```python
from build123d import *

# Parameters (mm, degrees)
SKETCH1_W                        = 69.85
SKETCH1_H                        = 838.2
BASE_FLANGE1_DEPTH               = 3.2639
EDGE_FLANGE2_STRIP_W             = 15.5956
EDGE_FLANGE2_STRIP_H             = 3.2639
EDGE_FLANGE2_STRIP_CUT_DEPTH     = 838.2
EDGE_FLANGE2_STRIP_2_W           = 15.5956
EDGE_FLANGE2_STRIP_2_H           = 3.2639
EDGE_FLANGE2_STRIP_CUT_2_DEPTH   = 838.2
EDGE_FLANGE2_DEPTH               = 838.2
EDGE_FLANGE2_BEND_DEPTH          = 838.2
SKETCH23_W                       = 101.6
SKETCH23_H                       = 34.925
BOSS_EXTRUDE1_DEPTH              = 3.2639
SKETCH24_W                       = 101.6
SKETCH24_H                       = 34.925
BOSS_EXTRUDE2_DEPTH              = 3.2639
SKETCH32_W                       = 88.9
SKETCH32_H                       = 34.925
BOSS_EXTRUDE3_DEPTH              = 3.2639
BOSS_EXTRUDE4_START              = -3.2639
SKETCH33_W                       = 88.9
SKETCH33_H                       = 34.925
BOSS_EXTRUDE4_DEPTH              = 3.2639
F_10_0_1935_DIAMETER_HOLE2_D     = 4.9149
LPATTERN2_COUNT                  = 4
LPATTERN2_PITCH                  = 155.575
F_25_64_0_39063_DIAMETER_HOLE1_D = 9.922002
F_10_0_1935_DIAMETER_HOLE3_D     = 4.9149
FILLET2_R                        = 6.35


# Sheet-metal steps are written as plain solids
with BuildPart() as part:
    # Sketch1 → Base-Flange1 (new body)
    with BuildSketch(Plane(origin=(0, 0, 0), x_dir=(1, 0, 0), z_dir=(0, 1, 0))):
        with Locations((0, 419.1)):
            Rectangle(SKETCH1_W, SKETCH1_H)
    extrude(amount=-BASE_FLANGE1_DEPTH)

    # Edge-Flange2 strip (across the edge) → Edge-Flange2 strip cut (cut)
    with BuildSketch(Plane(origin=(34.925, -3.2639, -838.2), x_dir=(-1, 0, 0), z_dir=(0, 0, 1))):
        with Locations((-3.2639, -1.63195)):
            Rectangle(EDGE_FLANGE2_STRIP_W, EDGE_FLANGE2_STRIP_H)
    extrude(amount=EDGE_FLANGE2_STRIP_CUT_DEPTH, mode=Mode.SUBTRACT)

    # Edge-Flange2 strip 2 (across the edge) → Edge-Flange2 strip cut 2 (cut)
    with BuildSketch(Plane(origin=(-34.925, -3.2639, 0), x_dir=(1, 0, 0), z_dir=(0, 0, -1))):
        with Locations((-3.2639, -1.63195)):
            Rectangle(EDGE_FLANGE2_STRIP_2_W, EDGE_FLANGE2_STRIP_2_H)
    extrude(amount=EDGE_FLANGE2_STRIP_CUT_2_DEPTH, mode=Mode.SUBTRACT)

    # Edge-Flange2 section (across the edge) → Edge-Flange2 (add)
    with BuildSketch(Plane(origin=(34.925, -3.2639, -838.2), x_dir=(-1, 0, 0), z_dir=(0, 0, 1))):
        with BuildLine():
            Line((0, 1.27), (0, 18.9611))
            Line((0, 18.9611), (3.2639, 18.9611))
            Line((3.2639, 18.9611), (3.2639, 1.27))
            ThreePointArc((3.2639, 1.27), (3.635874388, 0.371974388), (4.5339, 0))
            Line((4.5339, 0), (4.5339, -3.2639))
            ThreePointArc((4.5339, -3.2639), (1.327948565, -1.935951435), (0, 1.27))
        make_face()
    extrude(amount=EDGE_FLANGE2_DEPTH)

    # Edge-Flange2 section 2 (across the edge) → Edge-Flange2 bend (add)
    with BuildSketch(Plane(origin=(-34.925, -3.2639, 0), x_dir=(1, 0, 0), z_dir=(0, 0, -1))):
        with BuildLine():
            Line((0, 1.27), (0, 18.9611))
            Line((0, 18.9611), (3.2639, 18.9611))
            Line((3.2639, 18.9611), (3.2639, 1.27))
            ThreePointArc((3.2639, 1.27), (3.635874388, 0.371974388), (4.5339, 0))
            Line((4.5339, 0), (4.5339, -3.2639))
            ThreePointArc((4.5339, -3.2639), (1.327948565, -1.935951435), (0, 1.27))
        make_face()
    extrude(amount=EDGE_FLANGE2_BEND_DEPTH)

    # Sketch23 → Boss-Extrude1 (add)
    with BuildSketch(Plane.ZY.offset(34.925)):
        with Locations((-787.4, -39.6875)):
            Rectangle(SKETCH23_W, SKETCH23_H)
    extrude(amount=-BOSS_EXTRUDE1_DEPTH)

    # Sketch24 → Boss-Extrude2 (add)
    with BuildSketch(Plane(origin=(34.925, 0, 0), x_dir=(0, 0, -1), z_dir=(1, 0, 0))):
        with Locations((787.4, -39.6875)):
            Rectangle(SKETCH24_W, SKETCH24_H)
    extrude(amount=-BOSS_EXTRUDE2_DEPTH)

    # Sketch32 → Boss-Extrude3 (add)
    with BuildSketch(Plane.ZY.offset(34.925)):
        with Locations((-44.45, -39.6875)):
            Rectangle(SKETCH32_W, SKETCH32_H)
    extrude(amount=-BOSS_EXTRUDE3_DEPTH)

    # Sketch33 → Boss-Extrude4 (add)
    with BuildSketch(Plane(origin=(34.925, 0, 0), x_dir=(0, 0, -1), z_dir=(1, 0, 0)).offset(BOSS_EXTRUDE4_START)):
        with Locations((44.45, -39.6875)):
            Rectangle(SKETCH33_W, SKETCH33_H)
    extrude(amount=BOSS_EXTRUDE4_DEPTH)

    # #10 (0.1935) Diameter Hole2 (through all)
    with Locations(Plane.ZY.offset(34.925)):
        with Locations((-203.2, -14.2875)):
            f_10_0_1935_diameter_hole2 = Hole(F_10_0_1935_DIAMETER_HOLE2_D / 2)

    # LPattern2: #10 (0.1935) Diameter Hole2 ×4
    with Locations(*[(0, 0, -i * LPATTERN2_PITCH) for i in range(1, LPATTERN2_COUNT)]):
        add(f_10_0_1935_diameter_hole2, mode=Mode.SUBTRACT)

    # 25/64 (0.39063) Diameter Hole1 (through all)
    with Locations(Plane.ZY.offset(34.925)):
        with Locations((-825.5, -14.442948), (-825.5, -46.192948), (-749.3, -14.442948), (-749.3, -46.192948)):
            Hole(F_25_64_0_39063_DIAMETER_HOLE1_D / 2)

    # #10 (0.1935) Diameter Hole3 (through all)
    with Locations(Plane.ZY.offset(34.925)):
        with Locations((-82.55, -12.7), (-82.55, -50.8), (-6.35, -12.7), (-6.35, -50.8)):
            Hole(F_10_0_1935_DIAMETER_HOLE3_D / 2)

    # Fillet2
    fillet2_edges = [part.edges().sort_by_distance(p)[0] for p in [
        (-33.29305, -22.225, -88.9),
        (-33.29305, -57.15, -88.9),
        (-33.29305, -57.15, 0),
        (33.29305, -57.15, 0),
        (33.29305, -22.225, -88.9),
        (33.29305, -57.15, -88.9),
        (-33.29305, -57.15, -736.6),
        (-33.29305, -22.225, -736.6),
        (-33.29305, -57.15, -838.2),
        (33.29305, -57.15, -838.2),
        (33.29305, -57.15, -736.6),
        (33.29305, -22.225, -736.6),
    ]]
    fillet(fillet2_edges, radius=FILLET2_R)


solid = part.part
```
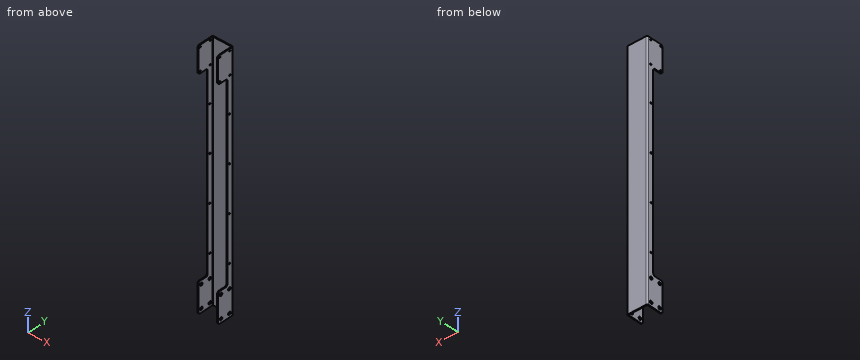
The listing builds one solid part. Answer for the finished solid, in the listing's coordinates (mm). Give positions to 0.01 mm unless a question says otherwise; leave off trailing zeros. Order: outer loops, then holes, each group sorted by start corner. A loop starts at its lowest first (then second) coordinate and runs counter-clockwise, first axis right, second up. Notation, with made-up numbers: (60, -18) -> (105, -18) arc R31 cw to (105, 12) -> close; hole circle Ø7 at (77.5, -30.5). An arc over 180 degrees is marked (long way). Write each question's results on one line, items separated by ' | '.
Q1. Straight lines are drawn through the part: probe 1 along X at (y, z) = (-14, -295) (3 decimals); probe 2 along Y at (x, z) = (33.5, -749.3); probe 3 along Y at (x, z) = (-25, -77.5). For each, find the intervals that lie inside material, in ascending order. Write a range as from..to.
Checked values:
probe 1: x = -34.925..-31.661, 31.661..34.925 | probe 2: y = -57.15..-51.15, -41.23..-19.4, -9.48..-1.23 | probe 3: y = -3.26..0
Q2. The part is cut by section B-B, the plane x = -19. Give the vertices of the cut face in (y, z), and give its area (3 significant figures).
Checked values:
outline: (-3.26, -838.2) -> (0, -838.2) -> (0, 0) -> (-3.26, 0) -> close | area: 2,740 mm^2
Q3. The part is cut by section A-A, the plane z = -610. Give the vertices of the cut face in (x, y) (3 decimals), and give its area (3 significant figures).
Checked values:
outline: (-34.925, -22.225) -> (-31.661, -22.225) -> (-31.661, -4.534) arc R1.27 cw to (-30.391, -3.264) -> (30.391, -3.264) arc R1.27 cw to (31.661, -4.534) -> (31.661, -22.225) -> (34.925, -22.225) -> (34.925, -4.534) arc R4.534 ccw to (30.391, 0) -> (-30.391, 0) arc R4.534 ccw to (-34.925, -4.534) -> close | area: 344 mm^2
Q4. Each of these flat-tipped pins is pushed along its axis until it touches: P1, Ø13, axis at y = -46.19, z = -749.3, coming from the -X side (3 decimals); P2, Ø1, axis at x = -34, z = -385.5, coming from the -Y side (3 decimals). Where does it stop, or does it pass through?
Checked values:
P1: stops at x = -34.925 | P2: stops at y = -22.225
